Design review of the part shown in the three views and the two pictorial views. Dimensions are in mm from the part's minimum x, y and z. Round coordinates to 2 decimals unless told otherwise and drop trailing zeros. Order: outer loops, then holes, each group sorted by start corner. A loop starts at its lowest first (then second) coordinate and runs counter-clockwise, first axis right, second up. Notation, with made-up numbers: (47.5, 21.25) -> (103.5, 21.25) arc R14 cw to (103.5, 36.25) -> close; hole circle Ø3 at (15.25, 62). An arc over 180 degrees is marked (long way). Put each result on its own line as item: value. Start each with the question number.
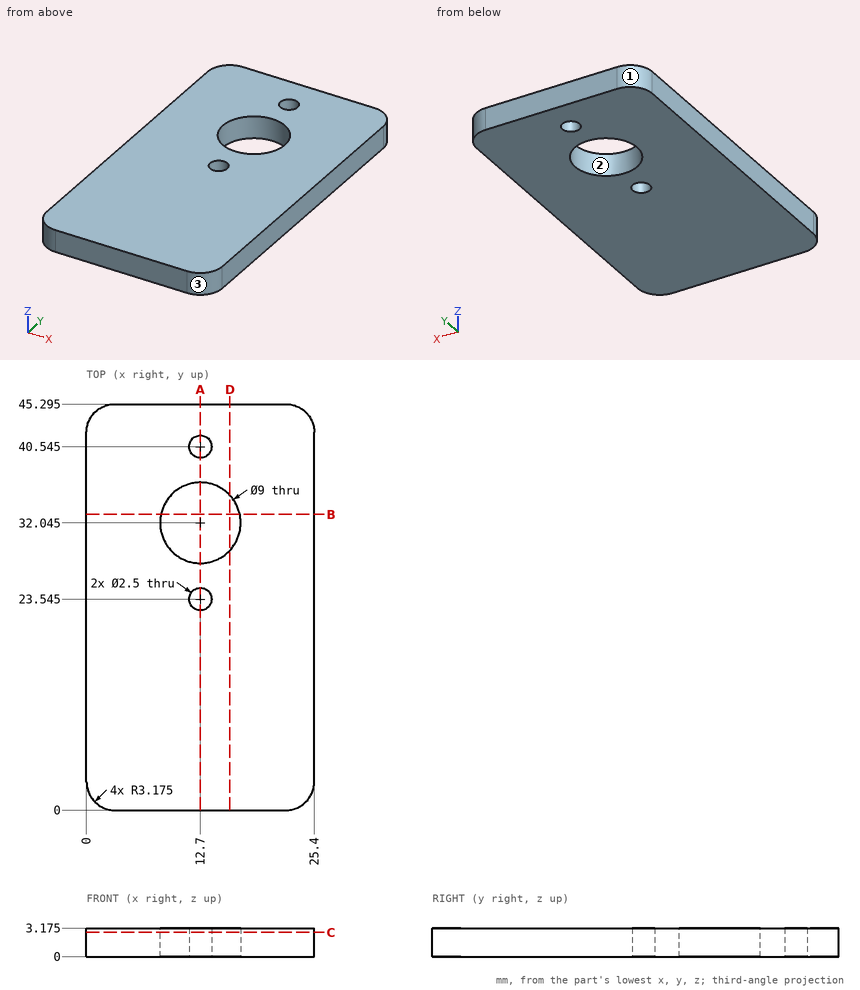
Q1. Wall thickness on probe 1 along Y at (x, z) = (12.7, 0.75) (3 decimals); probe 2 along X at (y, z) = (32, 1.3); probe 3 along Y at (x, z) = (11, 2.5) (3 decimals): over which ranges is each line inside the solid? List them lowest first. Write a range as [from, to].
Q2. Draft analysis for pull direction X (two halves, no side actions). For the marked faces 1, 2 and 3, state which applies: +X half, -X half, draft (parallel to the pull), parting line (faces both ways), or undercut.
Q3. Take a section at C-C on z = 2.7. Give the boundary of the cut face in (x, y) (3 decimals), and give its area (3 significant figures).
Q4. Take a section at A-A on x = 12.7. Give the boundary of the cut face in (y, z) (3 decimals), and give its area (3 significant figures).
Q5. Take a section at B-B on y = 33. Give the boundary of the cut face in (x, z) (1 decimal), and give its area (3 significant figures).
Q6. Take a section at D-D on x = 16. Give the boundary of the cut face in (y, z) (3 decimals), and give its area (3 significant figures).
Calculated:
1. probe 1: y = [0, 22.295], [24.795, 27.545], [36.545, 39.295], [41.795, 45.295]
1. probe 2: x = [0, 8.2], [17.2, 25.4]
1. probe 3: y = [0, 27.878], [36.212, 45.295]
2. face 1: -X half
2. face 2: undercut
2. face 3: +X half
3. outline: (0, 3.175) arc R3.175 ccw to (3.175, 0) -> (22.225, 0) arc R3.175 ccw to (25.4, 3.175) -> (25.4, 42.12) arc R3.175 ccw to (22.225, 45.295) -> (3.175, 45.295) arc R3.175 ccw to (0, 42.12) -> close; hole circle Ø9 at (12.7, 32.045); hole circle Ø2.5 at (12.7, 23.545); hole circle Ø2.5 at (12.7, 40.545)
3. area: 1,070 mm²
4. outline: (0, 0) -> (22.295, 0) -> (22.295, 3.175) -> (0, 3.175) -> close; (24.795, 0) -> (27.545, 0) -> (27.545, 3.175) -> (24.795, 3.175) -> close; (36.545, 0) -> (39.295, 0) -> (39.295, 3.175) -> (36.545, 3.175) -> close; (41.795, 0) -> (45.295, 0) -> (45.295, 3.175) -> (41.795, 3.175) -> close
4. area: 99.4 mm²
5. outline: (0, 0) -> (8.3, 0) -> (8.3, 3.2) -> (0, 3.2) -> close; (17.1, 0) -> (25.4, 0) -> (25.4, 3.2) -> (17.1, 3.2) -> close
5. area: 52.7 mm²
6. outline: (0, 0) -> (28.986, 0) -> (28.986, 3.175) -> (0, 3.175) -> close; (35.104, 0) -> (45.295, 0) -> (45.295, 3.175) -> (35.104, 3.175) -> close
6. area: 124 mm²
